from build123d import *

# Parameters (mm, degrees)
F0_R     = 6.35
F0_R_2   = 9.525
F1_DEPTH = 19.05


with BuildPart() as f1:
    # F0 (on Top) → F1 (new body)
    with BuildSketch(Plane.XY):
        with BuildLine():
            ThreePointArc((23.856802, 68.497253), (23.856237, 68.605633), (23.854543, 68.714001))
            ThreePointArc((23.854543, 68.714001), (13.685154, 78.892486), (3.082928, 69.165676))
            ThreePointArc((3.082928, 69.165676), (13.124727, 58.104941), (23.856802, 68.497253))
        make_face()
        with Locations((13.459112, 68.497253)):
            Circle(F0_R, mode=Mode.SUBTRACT)
        with BuildLine():
            ThreePointArc((-0.390204, 15.250903), (12.559621, 27.131474), (24.980767, 14.699216))
            Line((24.980767, 14.699216), (23.854543, 68.714001))
            ThreePointArc((23.854543, 68.714001), (23.856237, 68.605633), (23.856802, 68.497253))
            ThreePointArc((23.856802, 68.497253), (13.124727, 58.104941), (3.082928, 69.165676))
            Line((3.082928, 69.165676), (-0.390204, 15.250903))
        make_face()
        with BuildLine():
            ThreePointArc((-0.390204, 15.250903), (11.875102, 1.741044), (24.983527, 14.434475))
            ThreePointArc((24.983527, 14.434475), (24.982837, 14.566853), (24.980767, 14.699216))
            ThreePointArc((24.980767, 14.699216), (12.559621, 27.131474), (-0.390204, 15.250903))
        make_face()
        with Locations((12.283527, 14.434475)):
            Circle(F0_R_2, mode=Mode.SUBTRACT)
    extrude(amount=F1_DEPTH)


solid = f1.part
Work out the finished part from the listing and answer in its coordinate system (mm). Give positions to 0.01 mm unless a question says otherwise; leave off trailing zeros. Order: outer loops, then holes, each group sorted by start corner. A loop starts at its lowest first (then second) coordinate and runs counter-clockwise, first axis right, second up. Notation, with made-up numbers: (-18.75, -39) -> (-7.75, -39) arc R16 ccw to (-7.75, -31) -> close; hole circle Ø1 at (39, -36). An arc over 180 degrees is marked (long way). Answer as a JSON object with one key per item and string values. Group by question number.
1. Section C-C on z = 3 is taken. Determine the outline of the cut face in (x, y) (3 decimals), plus the area to 3 significant figures.
2. Flat-ended cylindrical pins translate along their axes: pin 1 Ø1.5 at (y, z) = (41, 10.5) entering from +X; pin 2 Ø10 at (y, z) = (55.5, 17) entering from +X; pin 3 Ø2 at (x, z) = (15, 10) entering from +Y; pin 4 Ø10 at (x, y) = (13.46, 68.5) entering from -Z. Find the tip coordinate at first contact, or state that the pin passes through.
3. Consider line 1 along Y through (x, z) = (17.5, 2.5); line 2 along Y through (x, z) = (12.5, 1.75); line 3 along X through (y, z) = (15, 2.75). Determine where each line is inside the solid, lowest interval first. Write a range as [from, to].
4. The mould has two halves that part along Y. Classify faces 1 (the flat face through (12, 41, 19.05)), 2 (the flat face through (1.37, 42.59, 9.39)), 3 (the cylindrical face through (10.219, 5.136, 9.392)): released by +Y, released by -Y, zero draft, split by the parting line, or undercut.
5. Section B-B on y = 70.5 is taken. Determine the outline of the cut face in (x, z).
6. Section D-D on x = 19 is taken. Determine the outline of the cut face in (y, z).
7. Section A-A on x = 8 is taken. Determine the outline of the cut face in (y, z).
Result sheet:
{
 "1": {"outline": "(-0.39, 15.251) arc R12.7 ccw (long way) to (24.984, 14.434) arc R12.698 ccw to (24.981, 14.699) -> (23.855, 68.714) arc R10.398 ccw to (3.083, 69.166) -> close; hole circle Ø19.05 at (12.284, 14.434); hole circle Ø12.7 at (13.459, 68.497)", "area": "1,260 mm^2"},
 "2": {"pin 1": "stops at x = 24.45", "pin 2": "stops at x = 24.23", "pin 3": "stops at y = 78.88", "pin 4": "passes through"},
 "3": {"line 1": "y = [2.86, 6.46], [22.4, 63.6], [73.4, 78.08]", "line 2": "y = [1.74, 4.91], [23.96, 62.22], [74.77, 78.85]", "line 3": "x = [-0.4, 2.78], [21.79, 24.97]"},
 "4": {"face 1": "zero draft", "face 2": "released by +Y", "face 3": "undercut"},
 "5": {"outline": "(3.26, 0) -> (7.43, 0) -> (7.43, 19.05) -> (3.26, 19.05) -> close; (19.49, 0) -> (23.66, 0) -> (23.66, 19.05) -> (19.49, 19.05) -> close"},
 "6": {"outline": "(3.66, 0) -> (7.68, 0) -> (7.68, 19.05) -> (3.66, 19.05) -> close; (21.19, 0) -> (65.4, 0) -> (65.4, 19.05) -> (21.19, 19.05) -> close; (71.6, 0) -> (77.3, 0) -> (77.3, 19.05) -> (71.6, 19.05) -> close"},
 "7": {"outline": "(2.48, 0) -> (5.93, 0) -> (5.93, 19.05) -> (2.48, 19.05) -> close; (22.94, 0) -> (65.25, 0) -> (65.25, 19.05) -> (22.94, 19.05) -> close; (71.74, 0) -> (77.35, 0) -> (77.35, 19.05) -> (71.74, 19.05) -> close"}
}
